Source: CAD feature listing. Evaluate the final solid. Frame: model axes, mm. Face numbers are marked on the shaded views. A direction names the side the tool comes from. Give positions to 0.01 mm unless a question says otherwise; leave off trailing zeros. Loops run counter-clockwise (first coordinate to the right, second up) from the corner with the lowest first, then second, coordinate; pieces in that order, holes last. Notation, with made-up numbers: (6, -31) -> (28, -31) arc R24 ccw to (28, -16) -> close; hole circle Ø10 at (-3.5, 16). An arc over 180 degrees is marked (long way). Return JSON: item names as keys, results as strings. Group by question number.
(1) Cut plane C-C on z = 14. Return loops of the section in (x, y), then the cut area to 3 significant figures.
(2) Pin query (flat end, axial travel): pin 1 (22 mm diameter, centred on x = -38.5, z = 15, fed in from +Y); pin 2 (2 mm diameter, centred on y = -2, z = 34.5, fed in from +X); pin 3 (22 mm diameter, centred on x = -3.5, z = 5, fed in from -Y). Return the tip coordinate at first contact, or that it passes through.
(3) Draft query along Z for the marked faces 3, 4, 5 and 6. Return one class per face: released by +Z, released by -Z, zero draft, split by the parting line, or undercut.
(4) Cut plane D-D on z = -17. Return loops of the section in (x, y), then the cut area to 3 significant figures.
(5) Ray query, line 1 (Z direction, x = -19.5, y = 4); line 2 (X direction, y = -1.25, z = 14.5); line 3 (Y direction, x = -3, z = -15). Return the intervals inside material, ascending. Write a range as from..to.
(6) Access query for the marked faces 1 and 2. Directions: +Z, -Z, +X, -X, +Y, -Y. A direction counts if a zero-diameter tool reaches every point of the face in a straight line with its end or side. Return the directions, or none.
(7) Cut plane A-A on y = -4.25. Return loops of the section in (x, z).
(8) Cut plane B-B on x = -40.5. Return loops of the section in (y, z), then the cut area to 3 significant figures.
```python
from build123d import *

# Parameters (mm, degrees)
BOSS_EXTRUDE1_DEPTH      = 12
BOSS_EXTRUDE1_DEPTH_BACK = 6
BOSS_EXTRUDE2_DEPTH      = 2.5


with BuildPart() as part:
    # Sketch1 → Boss-Extrude1 (new, two sides: drawn at the far end of the back side and taken through both)
    with BuildSketch(Plane(origin=(0, 0, 0), x_dir=(1, 0, 0), z_dir=(0, 1, 0)).offset(-BOSS_EXTRUDE1_DEPTH_BACK)):
        with BuildLine():
            Line((-77.044025157, 19.748427673), (-77.044025157, -30.251572327))
            ThreePointArc((-77.044025157, -30.251572327), (-72.650626875, -40.858174045), (-62.044025157, -45.251572327))
            Line((-62.044025157, -45.251572327), (37.955974843, -45.251572327))
            ThreePointArc((37.955974843, -45.251572327), (48.562576561, -40.858174045), (52.955974843, -30.251572327))
            Line((52.955974843, -30.251572327), (52.955974843, 19.748427673))
            ThreePointArc((52.955974843, 19.748427673), (48.562576561, 30.355029391), (37.955974843, 34.748427673))
            Line((37.955974843, 34.748427673), (-62.044025157, 34.748427673))
            ThreePointArc((-62.044025157, 34.748427673), (-72.650626875, 30.355029391), (-77.044025157, 19.748427673))
        make_face()
        with BuildLine():
            Line((-74.044025157, 19.748427673), (-74.044025157, -30.251572327))
            ThreePointArc((-74.044025157, -30.251572327), (-70.529306531, -38.736853701), (-62.044025157, -42.251572327))
            Line((-62.044025157, -42.251572327), (37.955974843, -42.251572327))
            ThreePointArc((37.955974843, -42.251572327), (46.441256217, -38.736853701), (49.955974843, -30.251572327))
            Line((49.955974843, -30.251572327), (49.955974843, 19.748427673))
            ThreePointArc((49.955974843, 19.748427673), (46.441256217, 28.233709047), (37.955974843, 31.748427673))
            Line((37.955974843, 31.748427673), (-62.044025157, 31.748427673))
            ThreePointArc((-62.044025157, 31.748427673), (-70.529306531, 28.233709047), (-74.044025157, 19.748427673))
        make_face(mode=Mode.SUBTRACT)
    extrude(amount=BOSS_EXTRUDE1_DEPTH + BOSS_EXTRUDE1_DEPTH_BACK)

    # Sketch1_3 → Boss-Extrude2 (add)
    with BuildSketch(Plane(origin=(0, 0, 0), x_dir=(1, 0, 0), z_dir=(0, 1, 0))):
        with BuildLine():
            ThreePointArc((-74.044025157, 19.748427673), (-70.529306531, 28.233709047), (-62.044025157, 31.748427673))
            Line((-62.044025157, 31.748427673), (37.955974843, 31.748427673))
            ThreePointArc((37.955974843, 31.748427673), (46.441256217, 28.233709047), (49.955974843, 19.748427673))
            Line((49.955974843, 19.748427673), (49.955974843, -30.251572327))
            ThreePointArc((49.955974843, -30.251572327), (46.441256217, -38.736853701), (37.955974843, -42.251572327))
            Line((37.955974843, -42.251572327), (-62.044025157, -42.251572327))
            ThreePointArc((-62.044025157, -42.251572327), (-70.529306531, -38.736853701), (-74.044025157, -30.251572327))
            Line((-74.044025157, -30.251572327), (-74.044025157, 19.748427673))
        make_face()
        with BuildLine():
            ThreePointArc((-51.159476074, -20.33614651), (-45.159476074, -26.33614651), (-39.159476074, -20.33614651))
            Line((-39.159476074, -20.33614651), (-39.159476074, 9.66385349))
            ThreePointArc((-39.159476074, 9.66385349), (-45.159476074, 15.66385349), (-51.159476074, 9.66385349))
            Line((-51.159476074, 9.66385349), (-51.159476074, -20.33614651))
        make_face(mode=Mode.SUBTRACT)
        with BuildLine():
            ThreePointArc((-30.207633374, -20.33614651), (-24.207633374, -26.33614651), (-18.207633374, -20.33614651))
            Line((-18.207633374, -20.33614651), (-18.207633374, 9.66385349))
            ThreePointArc((-18.207633374, 9.66385349), (-24.207633374, 15.66385349), (-30.207633374, 9.66385349))
            Line((-30.207633374, 9.66385349), (-30.207633374, -20.33614651))
        make_face(mode=Mode.SUBTRACT)
        with BuildLine():
            Line((27.07142576, 9.66385349), (27.07142576, -20.33614651))
            ThreePointArc((27.07142576, -20.33614651), (21.07142576, -26.33614651), (15.07142576, -20.33614651))
            Line((15.07142576, -20.33614651), (15.07142576, 9.66385349))
            ThreePointArc((15.07142576, 9.66385349), (21.07142576, 15.66385349), (27.07142576, 9.66385349))
        make_face(mode=Mode.SUBTRACT)
        with BuildLine():
            Line((6.119583059, 9.66385349), (6.119583059, -20.33614651))
            ThreePointArc((6.119583059, -20.33614651), (0.119583059, -26.33614651), (-5.880416941, -20.33614651))
            Line((-5.880416941, -20.33614651), (-5.880416941, 9.66385349))
            ThreePointArc((-5.880416941, 9.66385349), (0.119583059, 15.66385349), (6.119583059, 9.66385349))
        make_face(mode=Mode.SUBTRACT)
    extrude(amount=BOSS_EXTRUDE2_DEPTH)


solid = part.part
```
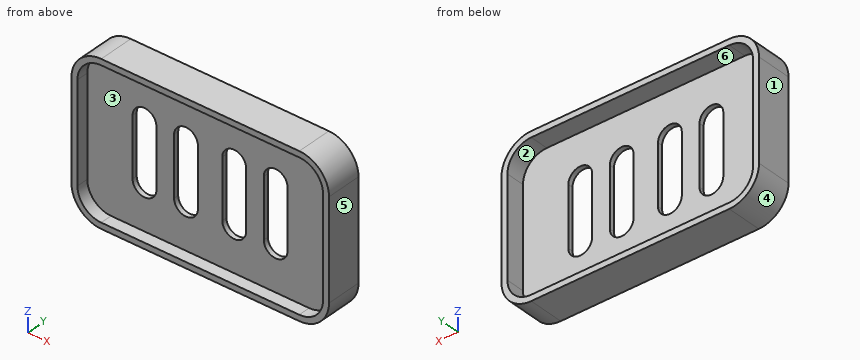
Answers:
{
 "1": {"outline": "(-77.04, -6) -> (-74.04, -6) -> (-74.04, 0) -> (-51.16, 0) -> (-51.16, 2.5) -> (-74.04, 2.5) -> (-74.04, 12) -> (-77.04, 12) -> close; (-39.16, 0) -> (-30.21, 0) -> (-30.21, 2.5) -> (-39.16, 2.5) -> close; (-18.21, 0) -> (-5.88, 0) -> (-5.88, 2.5) -> (-18.21, 2.5) -> close; (6.12, 0) -> (15.07, 0) -> (15.07, 2.5) -> (6.12, 2.5) -> close; (27.07, 0) -> (49.96, 0) -> (49.96, -6) -> (52.96, -6) -> (52.96, 12) -> (49.96, 12) -> (49.96, 2.5) -> (27.07, 2.5) -> close", "area": "298 mm²"},
 "2": {"pin 1": "y = 2.5", "pin 2": "x = 52.6", "pin 3": "y = 0"},
 "3": {"face 3": "undercut", "face 4": "released by -Z", "face 5": "zero draft", "face 6": "undercut"},
 "4": {"outline": "(-77.04, -6) -> (-74.04, -6) -> (-74.04, 0) -> (49.96, 0) -> (49.96, -6) -> (52.96, -6) -> (52.96, 12) -> (49.96, 12) -> (49.96, 2.5) -> (-74.04, 2.5) -> (-74.04, 12) -> (-77.04, 12) -> close", "area": "418 mm²"},
 "5": {"line 1": "-34.75..-31.75, 42.25..45.25", "line 2": "-77.04..-74.04, 49.96..52.96", "line 3": "0..2.5"},
 "6": {"face 1": "+Z, -Z, -X, +Y, -Y", "face 2": "+Y"},
 "7": {"outline": "(-77.04, -19.75) arc R15 ccw to (-62.04, -34.75) -> (37.96, -34.75) arc R15 ccw to (52.96, -19.75) -> (52.96, 30.25) arc R15 ccw to (37.96, 45.25) -> (-62.04, 45.25) arc R15 ccw to (-77.04, 30.25) -> close; hole (-74.04, -19.75) arc R12 ccw to (-62.04, -31.75) -> (37.96, -31.75) arc R12 ccw to (49.96, -19.75) -> (49.96, 30.25) arc R12 ccw to (37.96, 42.25) -> (-62.04, 42.25) arc R12 ccw to (-74.04, 30.25) -> close"},
 "8": {"outline": "(-6, -34.75) -> (12, -34.75) -> (12, -31.75) -> (2.5, -31.75) -> (2.5, -13.44) -> (0, -13.44) -> (0, -31.75) -> (-6, -31.75) -> close; (-6, 42.25) -> (0, 42.25) -> (0, 24.12) -> (2.5, 24.12) -> (2.5, 42.25) -> (12, 42.25) -> (12, 45.25) -> (-6, 45.25) -> close", "area": "199 mm²"}
}
